Autodesk Inventor part; units mm, degrees
ref_plane "XZ Plane" through (0, 0, 0) normal (0, 1, 0) x (-1, 0, 0)
ref_plane "XY Plane" through (0, 0, 0) normal (0, 0, 1) x (1, 0, 0)
sketch "Sketch1" plane through (0, 0, 0) normal (0, 0, 1) x (1, 0, 0)
  circle A0 centre (15, 0) radius 5
  line L0 (0, 0) -> (0, 7.4364)
  dimension "d0" = 10
  dimension "d2" = 15
revolve "Revolution1" add sketch "Sketch1" angle 360 about axis through (0, 0, 0) along (0, 1, 0)
ref_plane "Work Plane1" through (16, 0, 0) normal (1, 0, 0) x (0, 1, 0)
sketch "Sketch2" plane through (16, 0, 0) normal (1, 0, 0) x (0, 1, 0)
  circle A0 centre (0, 0) radius 3.175
  dimension "d5" = 6.35
extrude "Extrusion1" add sketch "Sketch2" along normal blind 25.4
mirror "Mirror1" about plane through (0, 0, 0) normal (1, 0, 0)
sketch "Sketch3" plane through (-16, 0, 0) normal (-1, 0, 0) x (0, 1, 0)
  circle A0 centre (0, 0) radius 3.175
  dimension "d8" = 6.35
extrude "Extrusion2" add sketch "Sketch3" along normal blind 152.4
ref_plane "Work Plane2" through (-16, 0, 0) normal (1, 0, 0) x (0, 1, 0)
properties part number "string manager prototype"
The model under review builds one solid part; all positions refer to its coordinate system, in mm. A direction names the side the tool comes from. Round coordinates to 2 decimals unless told otherwise and drop trailing zeros. Loops run counter-clockwise (first coordinate to the right, second up) from the corner with the lowest first, then second, coordinate; pieces in that order, holes last. Notation, with made-up numbers: (1, 9) - (47, 9) arc R34 ccw to (47, 40) - close; hole circle Ø8 at (-23.75, 70). An arc over 180 degrees is marked (long way). Use a Markdown table: item, result. Add a question column.
Q1. Add section B-B (y = 0). State the section outline as (x, z) points (3 decimals), plus the area to 3 significant figures.
Q2. Machinability: for faces 1 (the face through (-92.58, -0.69, -3.1)), 2 (the face through (29.97, -0.69, 3.1)), 3 (the face through (-168.4, 0, 0)), which of the approach directions +Z, -Z, +X, -X, +Y, -Y give a long, thin tool a straight path to every point of the face, cutting with its end or side? Answer none if there is none.
Q3. Insertion check: pin 1 Ø1 at (y, z) = (-0.5, 4) entering from +X (3 decimals); pin 2 Ø12 at (x, z) = (-24.5, 0.5) entering from +Y. Each pin has a flat end and moves straight along its axis. Give the tip position at first contact, or say it passes through.
Q4. Add section A-A (z = 0). State the section outline as (x, y) points (3 decimals), plus the area to 3 significant figures.
Q5. For probe 1 along X at (y, z) = (-2, -6); probe 2 along Z at (x, y) = (-137.5, -0.5); probe 3 along X at (y, z) = (4.25, -6.5), list the stretches that pass through material, from the lowest coordinate up.
Q6. Add section C-C (x = -136.5). State the section outline as (y, z) points (3 decimals).
Worked answers:
| question | item | result |
|---|---|---|
| 1 | outline | (-168.4, -3.175) - (-19.746, -3.175) arc R20 ccw to (19.746, -3.175) - (41.4, -3.175) - (41.4, 3.175) - (19.746, 3.175) arc R20 ccw to (-19.746, 3.175) - (-168.4, 3.175) - close; hole circle Ø20 at (0, 0) |
| 1 | area | 2,020 mm² |
| 2 | face 1 | -X |
| 2 | face 2 | +X |
| 2 | face 3 | +Z, -Z, -X, +Y, -Y |
| 3 | pin 1 | x = 19.675 |
| 3 | pin 2 | y = 3.57 |
| 4 | outline | (-168.4, -3.175) - (-18.863, -3.175) arc R5 ccw (long way) to (-18.863, 3.175) - (-168.4, 3.175) - close; (18.863, -3.175) - (41.4, -3.175) - (41.4, 3.175) - (18.863, 3.175) arc R5 ccw (long way) to start |
| 4 | area | 1,240 mm² |
| 5 | probe 1 | -18.64 to -8.52, 8.52 to 18.64 |
| 5 | probe 2 | -3.14 to 3.14 |
| 5 | probe 3 | -16.39 to -10.52, 10.52 to 16.39 |
| 6 | outline | circle Ø6.35 at (0, 0) |
